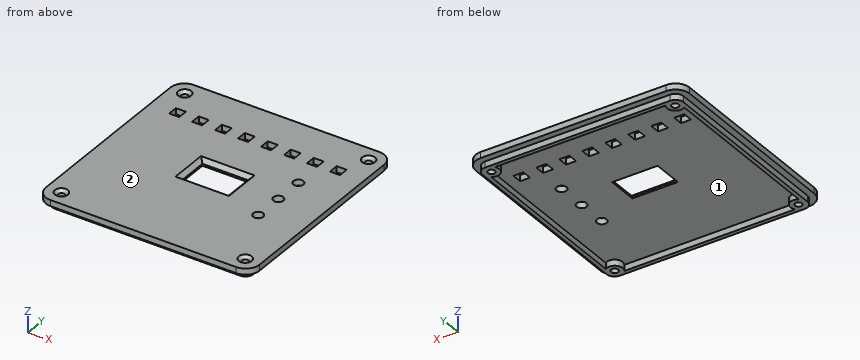
```python
from build123d import *
from build123d.topology import SkipClean

# Parameters (mm, degrees)
ESTRUSIONE_ESTRUSIONE1_DEPTH  = 3
TAGLIO_ESTRUSIONE1_REACH      = 105.055
SCHIZZO2_R                    = 1.75
SMUSSO1_SIZE                  = 1.5
SCHIZZO3_W                    = 22.789608278
SCHIZZO3_H                    = 15.099999313
TAGLIO_ESTRUSIONE2_DEPTH      = 104.055261945
SMUSSO2_SIZE                  = 2
SCHIZZO4_R                    = 1.75
ESTRUSIONE_ESTRUSIONE2_DEPTH  = 3
TAGLIO_ESTRUSIONE3_DEPTH      = 104.18617647
TAGLIO_ESTRUSIONE3_DEPTH_BACK = 104.18617647
SCHIZZO5_R                    = 2.5
SCHIZZO5_W                    = 5
SCHIZZO5_H                    = 5


with BuildPart() as part:
    # Schizzo1 → Estrusione-Estrusione1 (new body)
    with BuildSketch(Plane.XY.offset(126.00326253)):
        with BuildLine():
            Line((-77.628669492, 58.731382705), (15.346131117, 58.731382705))
            ThreePointArc((15.346131117, 58.731382705), (20.295878585, 56.681130173), (22.346131117, 51.731382705))
            Line((22.346131117, 51.731382705), (22.346131117, -41.243417905))
            ThreePointArc((22.346131117, -41.243417905), (20.295878585, -46.193165373), (15.346131117, -48.243417905))
            Line((15.346131117, -48.243417905), (-77.628669492, -48.243417905))
            ThreePointArc((-77.628669492, -48.243417905), (-82.578416961, -46.193165373), (-84.628669492, -41.243417905))
            Line((-84.628669492, -41.243417905), (-84.628669492, 51.731382705))
            ThreePointArc((-84.628669492, 51.731382705), (-82.578416961, 56.681130173), (-77.628669492, 58.731382705))
        make_face()
    extrude(amount=ESTRUSIONE_ESTRUSIONE1_DEPTH)

    # Schizzo2 → Taglio-Estrusione1 (cut, up to next)
    with BuildSketch(Plane.XY.offset(129.00326253), mode=Mode.PRIVATE) as taglio_estrusione1_sk1:
        with Locations((-77.141361898, 51.24407511)):
            Circle(SCHIZZO2_R)
    taglio_estrusione1_tool1 = extrude(taglio_estrusione1_sk1.sketch, amount=-TAGLIO_ESTRUSIONE1_REACH, mode=Mode.PRIVATE) & part.part
    # Schizzo2 → Taglio-Estrusione1 (cut, up to next)
    with BuildSketch(Plane.XY.offset(129.00326253), mode=Mode.PRIVATE) as taglio_estrusione1_sk2:
        with Locations((14.858823522, 51.24407511)):
            Circle(SCHIZZO2_R)
    taglio_estrusione1_tool2 = extrude(taglio_estrusione1_sk2.sketch, amount=-TAGLIO_ESTRUSIONE1_REACH, mode=Mode.PRIVATE) & part.part
    # Schizzo2 → Taglio-Estrusione1 (cut, up to next)
    with BuildSketch(Plane.XY.offset(129.00326253), mode=Mode.PRIVATE) as taglio_estrusione1_sk3:
        with Locations((14.858823522, -40.75611031)):
            Circle(SCHIZZO2_R)
    taglio_estrusione1_tool3 = extrude(taglio_estrusione1_sk3.sketch, amount=-TAGLIO_ESTRUSIONE1_REACH, mode=Mode.PRIVATE) & part.part
    # Schizzo2 → Taglio-Estrusione1 (cut, up to next)
    with BuildSketch(Plane.XY.offset(129.00326253), mode=Mode.PRIVATE) as taglio_estrusione1_sk4:
        with Locations((-77.128669492, -40.768617295)):
            Circle(SCHIZZO2_R)
    taglio_estrusione1_tool4 = extrude(taglio_estrusione1_sk4.sketch, amount=-TAGLIO_ESTRUSIONE1_REACH, mode=Mode.PRIVATE) & part.part
    add(taglio_estrusione1_tool1.solids().sort_by_distance((-77.141362, 51.244075, 129.003263))[0], mode=Mode.SUBTRACT)
    add(taglio_estrusione1_tool2.solids().sort_by_distance((14.858824, 51.244075, 129.003263))[0], mode=Mode.SUBTRACT)
    add(taglio_estrusione1_tool3.solids().sort_by_distance((14.858824, -40.75611, 129.003263))[0], mode=Mode.SUBTRACT)
    add(taglio_estrusione1_tool4.solids().sort_by_distance((-77.128669, -40.768617, 129.003263))[0], mode=Mode.SUBTRACT)

    # Smusso1
    smusso1_edges = [part.edges().sort_by_distance(p)[0] for p in [
        (-78.878669492, -40.768617295, 129.00326253),
        (13.108823522, -40.75611031, 129.00326253),
        (13.108823522, 51.24407511, 129.00326253),
        (-78.891361898, 51.24407511, 129.00326253),
    ]]
    chamfer(smusso1_edges, length=SMUSSO1_SIZE)

    # Schizzo3 → Taglio-Estrusione2 (cut, through all)
    with BuildSketch(Plane.XY.offset(129.00326253)):
        with Locations((-31.141270458, 5.263005749)):
            Rectangle(SCHIZZO3_W, SCHIZZO3_H)
    extrude(amount=-TAGLIO_ESTRUSIONE2_DEPTH, mode=Mode.SUBTRACT)

    # Smusso2
    smusso2_edges = [part.edges().sort_by_distance(p)[0] for p in [
        (-42.536074597, 5.263005749, 129.00326253),
        (-31.141270458, -2.286993907, 129.00326253),
        (-19.746466319, 5.263005749, 129.00326253),
        (-31.141270458, 12.813005406, 129.00326253),
    ]]
    chamfer(smusso2_edges, length=SMUSSO2_SIZE)

    # Schizzo4 → Estrusione-Estrusione2 (add)
    with SkipClean():  # the faces are left unmerged after this step: merging them gives an invalid solid
        with BuildSketch(Plane(origin=(0, 0, 126.00326253), x_dir=(-1, 0, 0), z_dir=(0, 0, -1))):
            with BuildLine():
                ThreePointArc((81.428669492, -41.043417905), (80.257096617, -43.87184503), (77.428669492, -45.043417905))
                Line((77.428669492, -45.043417905), (-15.146131117, -45.043417905))
                ThreePointArc((-15.146131117, -45.043417905), (-17.974558242, -43.87184503), (-19.146131117, -41.043417905))
                Line((-19.146131117, -41.043417905), (-19.146131117, 51.531382705))
                ThreePointArc((-19.146131117, 51.531382705), (-17.974558242, 54.359809829), (-15.146131117, 55.531382705))
                Line((-15.146131117, 55.531382705), (77.428669492, 55.531382705))
                ThreePointArc((77.428669492, 55.531382705), (80.257096617, 54.359809829), (81.428669492, 51.531382705))
                Line((81.428669492, 51.531382705), (81.428669492, -41.043417905))
            make_face()
            with Locations((77.128669492, -40.768617295)):
                Circle(SCHIZZO4_R, mode=Mode.SUBTRACT)
            with Locations((-14.858823522, 51.24407511)):
                Circle(SCHIZZO4_R, mode=Mode.SUBTRACT)
            with Locations((77.141361898, 51.24407511)):
                Circle(SCHIZZO4_R, mode=Mode.SUBTRACT)
            with Locations((-14.858823522, -40.75611031)):
                Circle(SCHIZZO4_R, mode=Mode.SUBTRACT)
            with BuildLine():
                Line((79.428669492, -37.496003661), (79.428669492, 47.940721611))
                ThreePointArc((79.428669492, 47.940721611), (74.300242368, 48.40295558), (73.838008399, 53.531382705))
                Line((73.838008399, 53.531382705), (-11.599070717, 53.531382705))
                ThreePointArc((-11.599070717, 53.531382705), (-12.042996434, 48.428248021), (-17.146131117, 47.984322305))
                Line((-17.146131117, 47.984322305), (-17.146131117, -37.496196748))
                ThreePointArc((-17.146131117, -37.496196748), (-12.042903383, -37.940190171), (-11.59890996, -43.043417905))
                Line((-11.59890996, -43.043417905), (73.838489834, -43.043417905))
                ThreePointArc((73.838489834, -43.043417905), (74.31112355, -37.929350689), (79.428669492, -37.496003661))
            make_face(mode=Mode.SUBTRACT)
        extrude(amount=ESTRUSIONE_ESTRUSIONE2_DEPTH)

    # Schizzo5 → Taglio-Estrusione3 (cut, two sides: drawn at the far end of the back side and taken through both)
    with SkipClean():  # the faces are left unmerged after this step: merging them gives an invalid solid
        with BuildSketch(Plane.XY.offset(129.00326253).offset(-TAGLIO_ESTRUSIONE3_DEPTH_BACK)):
            with Locations(Location((0.556781358, -9.75605951, 0), (0, 0, 180))):
                Circle(SCHIZZO5_R)
            with Locations(Location((0.556781358, 5.24397097, 0), (0, 0, 180))):
                Circle(SCHIZZO5_R)
            with Locations(Location((0.556781358, 20.24399891, 0), (0, 0, 180))):
                Circle(SCHIZZO5_R)
            with Locations((-71.391349259, 37.244047119)):
                Rectangle(SCHIZZO5_W, SCHIZZO5_H)
            with Locations((-59.891326399, 37.244047119)):
                Rectangle(SCHIZZO5_W, SCHIZZO5_H)
            with Locations((-48.391303539, 37.244047119)):
                Rectangle(SCHIZZO5_W, SCHIZZO5_H)
            with Locations((-36.891280679, 37.244047119)):
                Rectangle(SCHIZZO5_W, SCHIZZO5_H)
            with Locations((-25.391257819, 37.244047119)):
                Rectangle(SCHIZZO5_W, SCHIZZO5_H)
            with Locations((-13.891234958, 37.244047119)):
                Rectangle(SCHIZZO5_W, SCHIZZO5_H)
            with Locations((-2.391212098, 37.244047119)):
                Rectangle(SCHIZZO5_W, SCHIZZO5_H)
            with Locations((9.108810762, 37.244047119)):
                Rectangle(SCHIZZO5_W, SCHIZZO5_H)
        extrude(amount=TAGLIO_ESTRUSIONE3_DEPTH + TAGLIO_ESTRUSIONE3_DEPTH_BACK, mode=Mode.SUBTRACT)


solid = part.part
```
Check sheet for the modelled part. Datum: model origin and axes. Units: mm. Face numbers are marked on the shaded views. A direction names the side the tool comes from. Round coordinates to 2 decimals unless told otherwise and drop trailing zeros. Loops run counter-clockwise (first coordinate to the right, second up) from the corner with the lowest first, then second, coordinate; pieces in that order, holes last. Notation, with made-up numbers: M -14.75,-28 L 6.25,-28 A23 cw 6.25,-2 Z; hole C -39,-27.5 d6. An arc over 180 degrees is marked long. Answer as a JSON object with one key per item and string values.
1. Section check C-C (y = -23.5). Record the boundary of the cut face in (x, z).
Reply:
{"outline": "M -84.63,126 L -81.43,126 L -81.43,123 L -79.43,123 L -79.43,126 L 17.15,126 L 17.15,123 L 19.15,123 L 19.15,126 L 22.35,126 L 22.35,129 L -84.63,129 Z"}
2. Gauge pin test, flat ends, axial feed: P1, Ø0.9, axis at x = -39.5, z = 124.5, coming from the +Y side; P2, Ø3, axis at x = 14.86, y = -40.76, coming from the +Z side; P3, Ø6, axis at x = -49, y = 23.5, coming from the -Z side; P4, Ø2, axis at y = -11, z = 124, coming from the +X side. Record the tip position at first contact, or that the pin passes through.
Reply:
{"P1": "stops at y = 55.53", "P2": "passes through", "P3": "stops at z = 126", "P4": "stops at x = 19.15"}
3. Section check A-A (x = -25). Record the boundary of the cut face in (y, z), plus the area to 3 significant figures.
Reply:
{"outline": "M -48.24,126 L -45.04,126 L -45.04,123 L -43.04,123 L -43.04,126 L -2.29,126 L -2.29,127 L -4.29,129 L -48.24,129 Z; M 12.81,126 L 34.74,126 L 34.74,129 L 14.81,129 L 12.81,127 Z; M 39.74,126 L 53.53,126 L 53.53,123 L 55.53,123 L 55.53,126 L 58.73,126 L 58.73,129 L 39.74,129 Z", "area": "269 mm²"}
4. Access from +Z, -Z, +X, -X, +Y, -Y to the whole of each face (thin tool, end or side, straight path). Record for the marked faces 1 and 2.
Reply:
{"face 1": "-Z", "face 2": "+Z, +X, -X, +Y, -Y"}
5. Section check B-B (x = 9.5). Record the boundary of the cut face in (y, z), plus the area to 3 significant figures.
Reply:
{"outline": "M -48.24,126 L -45.04,126 L -45.04,123 L -43.04,123 L -43.04,126 L 34.74,126 L 34.74,129 L -48.24,129 Z; M 39.74,126 L 53.53,126 L 53.53,123 L 55.53,123 L 55.53,126 L 58.73,126 L 58.73,129 L 39.74,129 Z", "area": "318 mm²"}
6. Scan lines: line 1 (X direction, y = 51, z = 124.1); line 2 (Y direction, x = -4, z = 123.95); line 3 (Y direction, x = 13, z = 128.1). Record each from-to range of solid material in increasing order.
Reply:
{"line 1": "x = -81.43 to -78.87, -75.41 to -73.13, 10.88 to 13.13, 16.59 to 19.15", "line 2": "y = -45.04 to -43.04, 53.53 to 55.53", "line 3": "y = -48.24 to -42.19, -39.32 to 49.81, 52.68 to 58.73"}
